```python
from build123d import *

# Parameters (mm, degrees)
ESQUISSE1_R        = 1
ESQUISSE1_W        = 5
ESQUISSE1_H        = 5
ESQUISSE1_W_2      = 49
ESQUISSE1_H_2      = 36
BOSS_EXTRU_1_DEPTH = 5
CONG_1_R           = 2


with BuildPart() as part:
    # Esquisse1 → Boss.-Extru.1 (new body)
    with BuildSketch(Plane.XY):
        Polygon((0, 0), (7.5, 0), (7.5, -5), (12.5, -5), (12.5, 0), (58.5, 0), (58.5, -5), (63.5, -5), (63.5, 0), (71, 0), (81, 0), (81, 50), (71, 50), (0, 50), (0, 42.5), (-5, 42.5), (-5, 37.5), (0, 37.5), (0, 12.5), (-5, 12.5), (-5, 7.5), (0, 7.5), align=None)
        with Locations((6, 41)):
            Circle(ESQUISSE1_R, mode=Mode.SUBTRACT)
        with Locations((73.5, 10)):
            Rectangle(ESQUISSE1_W, ESQUISSE1_H, mode=Mode.SUBTRACT)
        with Locations((73.5, 40)):
            Rectangle(ESQUISSE1_W, ESQUISSE1_H, mode=Mode.SUBTRACT)
        with Locations((39, 25)):
            Rectangle(ESQUISSE1_W_2, ESQUISSE1_H_2, mode=Mode.SUBTRACT)
    extrude(amount=BOSS_EXTRU_1_DEPTH)

    # Congé1
    cong_1_edges = [part.edges().sort_by_distance(p)[0] for p in [
        (0, 50, 2.5),
        (81, 50, 2.5),
        (81, 0, 2.5),
        (0, 0, 2.5),
    ]]
    fillet(cong_1_edges, radius=CONG_1_R)


solid = part.part
```
Work out the finished part from the listing and answer in its coordinate system (mm). A direction names the side the tool comes from. Coordinates: 2 decimals unless noted, no trailing zeros. Write each loop counter-clockwise with the first axis right and the second up, starting at its lowest first coordinate (ties: lowest second). Pieces come first, ordered by that corner, then holes.
Q1. Which of the six approach directions +Z, -Z, +X, -X, +Y, -Y give full straight-line access (tool end or side, diameter ignored) to faces 4 (the face through (-2, 12.5, 2)), 5 (the face through (5, 0, 2)), 6 (the face through (63.5, -3, 2)), 7 (the face through (-2, 42.5, 2))?
Q2. A cutting plane is placed at A-A, the plane x = 6. Give the vertices of the cut face in (y, z), then the cut area to 3 significant figures.
Q3. Find the intervals of material crossed by line 1 (Y direction, x = 60.5, z = 1.1); line 2 (X direction, y = -2, z = 4.2); line 3 (Y direction, x = 6, z = 2.3), in increasing order.
Q4. A cutting plane is placed at B-B, the plane y = 11. Give the vertices of the cut face in (x, z).
Q5. A cutting plane is placed at C-C, the plane y = 41. Give the vertices of the cut face in (x, z).
Q6. Determine the mould class of faces 1 (the face through (76, 40, 2)), 2 (the face through (-5, 40, 2)), 3 (the face through (80.43, 49.4, 2.54)) for opening direction Y: released by +Y, released by -Y, zero draft, split by the parting line, or undercut.
Q7. A cutting plane is placed at D-D, the plane x = 61. Give the vertices of the cut face in (y, z).
Q8. Each of these flat-tipped pins is pushed along its axis until it touches: pin 1 Ø1 at (x, z) = (26, 1) entering from -Y; pin 2 Ø10 at (x, y) = (49.5, 9.5) entering from -Z; pin 3 Ø1.5 at (y, z) = (-2.5, 2.5) entering from +X; pin 4 Ø2.5 at (x, z) = (-3.5, 2.5) entering from -Y. Where does it stop, or does it pass through?
Findings below:
1. face 4: +Z, -Z, -X
1. face 5: +Z, -Z, -X, -Y
1. face 6: +Z, -Z, +X, -Y
1. face 7: +Z, -Z, -X, +Y
2. outline: (0, 0) - (40, 0) - (40, 5) - (0, 5) - close; (42, 0) - (50, 0) - (50, 5) - (42, 5) - close
2. area: 240 mm2
3. line 1: y = -5 to 7, 43 to 50
3. line 2: x = 7.5 to 12.5, 58.5 to 63.5
3. line 3: y = 0 to 40, 42 to 50
4. outline: (-5, 0) - (14.5, 0) - (14.5, 5) - (-5, 5) - close; (63.5, 0) - (71, 0) - (71, 5) - (63.5, 5) - close; (76, 0) - (81, 0) - (81, 5) - (76, 5) - close
5. outline: (-5, 0) - (5, 0) - (5, 5) - (-5, 5) - close; (7, 0) - (14.5, 0) - (14.5, 5) - (7, 5) - close; (63.5, 0) - (71, 0) - (71, 5) - (63.5, 5) - close; (76, 0) - (81, 0) - (81, 5) - (76, 5) - close
6. face 1: undercut
6. face 2: zero draft
6. face 3: released by +Y
7. outline: (-5, 0) - (7, 0) - (7, 5) - (-5, 5) - close; (43, 0) - (50, 0) - (50, 5) - (43, 5) - close
8. pin 1: stops at y = 0
8. pin 2: stops at z = 0
8. pin 3: stops at x = 63.5
8. pin 4: stops at y = 7.5
